```python
from build123d import *

# Parameters (mm, degrees)
SKETCH_1_R               = 11
EXTRUDE_1_DEPTH          = 28
SKETCH_2_R               = 14
EXTRUDE_2_DEPTH          = 12
FILLET_1_R               = 1
CHAMFER_1_SIZE           = 0.5
SKETCH_4_W               = 0.5
SKETCH_4_H               = 0.5
SKETCH_5_R               = 9
CUT_EXTRUDE_1_DEPTH      = 29
SKETCH_6_R               = 3
CUT_EXTRUDE_2_DEPTH      = 5
CUT_EXTRUDE_3_DEPTH      = 10.5
CUT_EXTRUDE_3_DEPTH_BACK = 2.2
CUT_EXTRUDE_3_START      = 28
SKETCH_7_W               = 42.252524986
SKETCH_7_H               = 12.607828389
SKETCH_8_R               = 1.5
CUT_EXTRUDE_4_DEPTH      = 10.5
SKETCH_8_3_R             = 1.5
CUT_EXTRUDE_5_DEPTH      = 54.724603976
CUT_EXTRUDE_START        = -7
SKETCH_9_R               = 2.75
CUT_EXTRUDE_6_DEPTH      = 10.5


with BuildPart() as part:
    # 草图1 → 凸台-拉伸1 (new body)
    with BuildSketch(Plane(origin=(0, 0, 0), x_dir=(1, 0, 0), z_dir=(0, 1, 0))):
        with Locations(Location((0, 0, 0), (0, 0, 270))):
            Circle(SKETCH_1_R)
    extrude(amount=EXTRUDE_1_DEPTH)

    # 草图2 → 凸台-拉伸2 (add)
    with BuildSketch(Plane(origin=(0, 28, 0), x_dir=(1, 0, 0), z_dir=(0, 1, 0))):
        with Locations(Location((0, 0, 0), (0, 0, 270))):
            Circle(SKETCH_2_R)
    extrude(amount=EXTRUDE_2_DEPTH)

    # 草图3 → 旋转1 (revolve)
    with BuildSketch(Plane.XY, mode=Mode.PRIVATE) as revolve_1_sk:
        with BuildLine():
            Line((-14, 40), (0, 40))
            Line((0, 40), (0, 45.445934077))
            ThreePointArc((0, 45.445934077), (-0.378215042, 45.409846851), (-0.742781353, 45.302887459))
            Line((-0.742781353, 45.302887459), (-14, 40))
        make_face()
    revolve(revolve_1_sk.sketch.rotate(Axis((0, 0, 0), (0, 1, 0)), 270), axis=Axis((0, 0, 0), (0, 1, 0)))

    # 圆角1
    fillet_1_edges = [part.edges().sort_by_distance(p)[0] for p in [
        (-14, 40, 0),
    ]]
    fillet(fillet_1_edges, radius=FILLET_1_R)

    # 倒角1
    chamfer_1_edges = [part.edges().sort_by_distance(p)[0] for p in [
        (0, 0, -11),
        (0, 28, -14),
    ]]
    chamfer(chamfer_1_edges, length=CHAMFER_1_SIZE)

    # 草图4 → 切除-旋转1 (revolve, cut)
    with BuildSketch(Plane(origin=(0, 0, 0), x_dir=(0, 0, -1), z_dir=(1, 0, 0)), mode=Mode.PRIVATE) as cut_revolve_1_sk:
        with Locations((-10.75, 25.75)):
            Rectangle(SKETCH_4_W, SKETCH_4_H)
        with Locations((-10.75, 22.65)):
            Rectangle(SKETCH_4_W, SKETCH_4_H)
        with Locations((-10.75, 19.55)):
            Rectangle(SKETCH_4_W, SKETCH_4_H)
        with Locations((-10.75, 16.45)):
            Rectangle(SKETCH_4_W, SKETCH_4_H)
        with Locations((-10.75, 13.35)):
            Rectangle(SKETCH_4_W, SKETCH_4_H)
        with Locations((-10.75, 10.25)):
            Rectangle(SKETCH_4_W, SKETCH_4_H)
        with Locations((-10.75, 7.15)):
            Rectangle(SKETCH_4_W, SKETCH_4_H)
        with Locations((-10.75, 4.05)):
            Rectangle(SKETCH_4_W, SKETCH_4_H)
    revolve(cut_revolve_1_sk.sketch.rotate(Axis((0, 0, 0), (0, 1, 0)), 180), axis=Axis((0, 0, 0), (0, 1, 0)), mode=Mode.SUBTRACT)

    # 草图5 → 切除-拉伸1 (cut)
    with BuildSketch(Plane.XZ):
        with Locations(Location((0, 0, 0), (0, 0, 270))):
            Circle(SKETCH_5_R)
    extrude(amount=-CUT_EXTRUDE_1_DEPTH, mode=Mode.SUBTRACT)

    # 草图6 → 切除-拉伸2 (cut)
    with BuildSketch(Plane.XZ.offset(-29)):
        with Locations(Location((0, 0, 0), (0, 0, 270))):
            Circle(SKETCH_6_R)
    extrude(amount=-CUT_EXTRUDE_2_DEPTH, mode=Mode.SUBTRACT)

    # 草图7 → 切除-拉伸3 (cut, two sides: drawn at the far end of the back side and taken through both)
    with BuildSketch(Plane(origin=(0, 0, 0), x_dir=(1, 0, 0), z_dir=(0, 1, 0)).offset(CUT_EXTRUDE_3_START - CUT_EXTRUDE_3_DEPTH_BACK)):
        with Locations((-1.165830539, -17.303914195)):
            Rectangle(SKETCH_7_W, SKETCH_7_H)
    extrude(amount=CUT_EXTRUDE_3_DEPTH + CUT_EXTRUDE_3_DEPTH_BACK, mode=Mode.SUBTRACT)

    # 草图8 → 切除-拉伸4 (cut)
    with BuildSketch(Plane.XY.offset(11)):
        with Locations((0, 32.3)):
            Circle(SKETCH_8_R)
    extrude(amount=-CUT_EXTRUDE_4_DEPTH, mode=Mode.SUBTRACT)

    # 草图8<3> → 切除-拉伸5 (cut, through all)
    with BuildSketch(Plane.XY.offset(11)):
        with Locations((-5, 32.3)):
            Circle(SKETCH_8_3_R)
        with Locations((5, 32.3)):
            Circle(SKETCH_8_3_R)
    extrude(amount=-CUT_EXTRUDE_5_DEPTH, mode=Mode.SUBTRACT)

    # 草图9 → 切除-拉伸6 (cut)
    with BuildSketch(Plane.XY.offset(CUT_EXTRUDE_START)):
        with Locations((5, 32.3)):
            Circle(SKETCH_9_R)
        with Locations((-5, 32.3)):
            Circle(SKETCH_9_R)
    extrude(amount=-CUT_EXTRUDE_6_DEPTH, mode=Mode.SUBTRACT)


solid = part.part
```
Work out the finished part from the listing and answer in its coordinate system (mm). A direction names the side the tool comes from. Coordinates: 2 decimals unless noted, no trailing zeros. Write each loop counter-clockwise with the first axis right and the second up, starting at its lowest first coordinate (ties: lowest second). Pieces come first, ordered by that corner, then holes.
Q1. A cutting plane is placed at C-C, the plane y = 8. Give the vertices of the cut face in (x, z).
Q2. A cutting plane is placed at A-A, the plane y = 32.3. Give the vertices of the cut face in (x, z).
Q3. Determine the mould class of faces 6 (the face through (-10.74, 2.13, -2.38)), 7 (the face through (0, 34, 11)), 8 (the face through (0.9, 31.46, -2.86)) for opening direction X: released by +X, released by -X, zero draft, split by the parting line, or undercut.
Q4. A cutting plane is placed at B-B, the plane z = 0. State how many separate pieces and enclosed holes the cut face has, then the cut area to 3 significant figures.
Q5. Which of the six approach directions +Z, -Z, +X, -X, +Y, -Y give full straight-line access (tool end or side, diameter ignored) to faces 1 (the face through (0, 38.5, 12)), 2 (the face through (-0.195, 33.787, 6.858)), 3 (the face through (0, 34, 0)), 4 (the face through (6.2, 31.1, -7)), 5 (the face through (4, 22.4, -10))?
Q6. Find the intervals of material crossed by line 1 (X direction, y = 32.3, z = -9); line 2 (X direction, y = 14.75, z = 0); line 3 (X direction, y = 4, z = -4), in increasing order.
Q7. Each of these flat-tipped pins is pushed along its axis until it touches: pin 1 Ø6.5 at (x, z) = (1, -1.5) entering from +Y; pin 2 Ø1 at (x, z) = (-4, 6) entering from +Y; pin 3 Ø12 at (y, z) = (21.5, -6.5) entering from -X; pin 4 Ø3 at (x, z) = (2.5, 4) entering from +Y. Where does it stop, or does it pass through?
Findings below:
1. outline: circle Ø22 at (0, 0); hole circle Ø18 at (0, 0)
2. outline: (-8.66, 11) arc R14 ccw to (-7.75, -11.66) - (-7.75, -7) - (-6.5, -7) - (-6.5, 11) - close; (-3.5, -7) - (-2.25, -7) - (-2.25, -13.82) arc R14 ccw to (2.25, -13.82) - (2.25, -7) - (3.5, -7) - (3.5, 11) - (1.5, 11) - (1.5, 2.6) arc R3 cw (long way) to (-1.5, 2.6) - (-1.5, 11) - (-3.5, 11) - close; (6.5, -7) - (7.75, -7) - (7.75, -11.66) arc R14 ccw to (8.66, 11) - (6.5, 11) - close
3. face 6: split by the parting line
3. face 7: zero draft
3. face 8: undercut
4. separate pieces: 1
4. enclosed holes: 2
4. area: 460 mm2
5. face 1: +Z, +X, -X, -Y
5. face 2: +Z
5. face 3: -Y
5. face 4: -Z
5. face 5: none
6. line 1: x = -10.72 to -7.75, -2.25 to 2.25, 7.75 to 10.72
6. line 2: x = -11 to -9, 9 to 11
6. line 3: x = -9.71 to -8.06, 8.06 to 9.71
7. pin 1: stops at y = 45.45
7. pin 2: stops at y = 42.92
7. pin 3: stops at x = -10.99
7. pin 4: stops at y = 44.31
